```python
from build123d import *

# Parameters (mm, degrees)
SKETCH1_W           = 21
SKETCH1_H           = 9
BOSS_EXTRUDE1_DEPTH = 410
SKETCH2_W           = 19
SKETCH2_H           = 408
CUT_EXTRUDE1_DEPTH  = 8
CUT_EXTRUDE2_DEPTH  = 8
SKETCH5_W           = 1
SKETCH5_H           = 8
CUT_EXTRUDE3_DEPTH  = 1
SKETCH6_W           = 1
SKETCH6_H           = 8
CUT_EXTRUDE4_DEPTH  = 1


with BuildPart() as part:
    # Sketch1 → Boss-Extrude1 (new body)
    with BuildSketch(Plane.XY):
        with Locations((10.5, -4.5)):
            Rectangle(SKETCH1_W, SKETCH1_H)
    extrude(amount=BOSS_EXTRUDE1_DEPTH)

    # Sketch2 → Cut-Extrude1 (cut)
    with BuildSketch(Plane(origin=(0, 0, 0), x_dir=(1, 0, 0), z_dir=(0, 1, 0))):
        with Locations((10.5, -205)):
            Rectangle(SKETCH2_W, SKETCH2_H)
    extrude(amount=-CUT_EXTRUDE1_DEPTH, mode=Mode.SUBTRACT)

    # Sketch4 → Cut-Extrude2 (cut)
    with BuildSketch(Plane(origin=(0, 0, 0), x_dir=(-1, 0, 0), z_dir=(0, 0, -1))):
        with BuildLine():
            Line((-20, -8.061503552), (-20, 0))
            Line((-20, 0), (-13.682887931, 0))
            ThreePointArc((-13.682887931, 0), (-18.014044946, -3.111884501), (-20, -8.061503552))
        make_face()
        with BuildLine():
            Line((-1, 0), (-7.317112069, 0))
            ThreePointArc((-7.317112069, 0), (-2.985955054, -3.111884501), (-1, -8.061503552))
            Line((-1, -8.061503552), (-1, 0))
        make_face()
    extrude(amount=-CUT_EXTRUDE2_DEPTH, mode=Mode.SUBTRACT)

    # Sketch5 → Cut-Extrude3 (cut)
    with BuildSketch(Plane(origin=(21, 0, 0), x_dir=(0, 0, -1), z_dir=(1, 0, 0))):
        with Locations((-0.5, -4)):
            Rectangle(SKETCH5_W, SKETCH5_H)
    extrude(amount=-CUT_EXTRUDE3_DEPTH, mode=Mode.SUBTRACT)

    # Sketch6 → Cut-Extrude4 (cut)
    with BuildSketch(Plane.ZY):
        with Locations((0.5, -4)):
            Rectangle(SKETCH6_W, SKETCH6_H)
    extrude(amount=-CUT_EXTRUDE4_DEPTH, mode=Mode.SUBTRACT)


solid = part.part
```
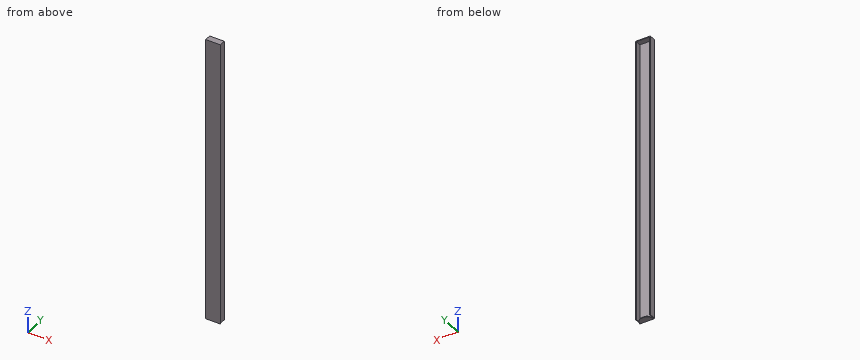
Verification items for the finished model (mm, model axes). Coordinates: 2 decimals unless noted, no trailing zeros. Order: outer loops, then holes, each group sorted by start corner. A loop starts at its lowest first (then second) coordinate and runs counter-clockwise, first axis right, second up. Notation, with made-up numbers: (80, -10.5) -> (130, -10.5) arc R19 ccw to (130, -1.5) -> close; hole circle Ø11 at (-30.75, 7). An arc over 180 degrees is marked (long way). Answer as CSV lines item,"result". Start each with the question number.
1) Gauge pin test, flat ends, axial feed: pin 1 Ø0.8 at (x, z) = (0.5, 0.5) entering from +Y; pin 2 Ø0.5 at (x, y) = (0.5, -3) entering from -Z. Record the tip position at first contact, or that the pin passes through.
2) Cross-section at B-B, the plane z = 359. Record the boundary of the cut face in (x, y).
3) Cross-section at A-A, the plane y = -4. Record the boundary of the cut face in (x, z).
4) Material ranges on L1, parallel to X at y = -3, z = 315; L2, parallel to Z at x = 6, y = -7.5; L3, parallel to Y at x = 12, z = 305.5, recorded low to high. Write a range as [from, to].
Conclusion:
1,pin 1,"stops at y = -8"
1,pin 2,"stops at z = 1"
2,outline,"(0, -9) -> (21, -9) -> (21, 0) -> (20, 0) -> (20, -8) -> (1, -8) -> (1, 0) -> (0, 0) -> close"
3,outline,"(0, 1) -> (1, 1) -> (1, 409) -> (20, 409) -> (20, 1) -> (21, 1) -> (21, 410) -> (0, 410) -> close; (2.37, 0) -> (18.63, 0) -> (18.63, 1) -> (2.37, 1) -> close"
4,L1,"x = [0, 1], [20, 21]"
4,L2,"z = [0, 1], [409, 410]"
4,L3,"y = [-9, -8]"
